Here's how the part is built. I have some questions about the finished solid (model axes, mm). Face numbers are marked on the shaded views. A direction names the side the tool comes from. Coordinates: 2 decimals unless noted, no trailing zeros. Write each loop counter-clockwise with the first axis right and the second up, starting at its lowest first coordinate (ties: lowest second). Pieces come first, ordered by that corner, then holes.
(1) Imagine slicing it at B-B, the plane z = -8.5. List the corners of the cut face in (x, y) for me, plus the area to 3 significant figures.
(2) Please list where these lines run through material, in increasing order: probe 1 along Y at (x, z) = (0, -6); probe 2 along X at (y, z) = (0, -9); probe 3 along X at (y, z) = (0, -7).
(3) Thinking about a two-plate mould opening in Y: for the marked faces 4, 5 and 6, which applies, released by +Y, released by -Y, zero draft, split by the parting line, or undercut?
(4) Which directions (+Z, -Z, +X, -X, +Y, -Y) give clear straight access to the entire face, cutting with the end or side of a thin tool? Please do the marked faces 1, 2 and 3.
(5) Imagine slicing it at A-A, the plane x = 0. List the corners of the cut face in (y, z) for me.
(6) For pin 1 Ø1 at (y, z) = (-4, -7.5) entering from +X; pin 2 Ø2 at (x, y) = (-3.5, 3) entering from +Z, each with a flat end and sliding along its axis, tell me the tip position at first contact or that it passes through.
(7) Imagine slicing it at C-C, the plane z = -1.5. List the corners of the cut face in (x, y) for me.
(8) Imagine slicing it at D-D, the plane z = -4.5. List the corners of the cut face in (x, y) for me, plus the area to 3 significant figures.
```python
from build123d import *

# Parameters (mm, degrees)
F1_R     = 9.1
F1_R_2   = 6.1
F2_DEPTH = 5
F3_DEPTH = 12
F3_TAPER = 12
F4_R     = 4.25
F4_R_2   = 2.75
F5_DEPTH = 10
F6_SIZE  = 2.5


with BuildPart() as f2:
    # F1 (on Top) → F2 (new body)
    with BuildSketch(Plane.XY):
        Circle(F1_R)
        Circle(F1_R_2, mode=Mode.SUBTRACT)
    extrude(amount=F2_DEPTH)

    # F1 (on Top) → F3 (join)
    with BuildSketch(Plane.XY):
        Circle(F1_R)
        Circle(F1_R_2, mode=Mode.SUBTRACT)
        Circle(F1_R_2)
    extrude(amount=-F3_DEPTH, taper=F3_TAPER)

    # F4 (on face) → F5 (cut)
    with BuildSketch(Plane(origin=(0, 0, -12), x_dir=(1, 0, 0), z_dir=(0, 0, -1))):
        Circle(F4_R)
        Circle(F4_R_2, mode=Mode.SUBTRACT)
    extrude(amount=-F5_DEPTH, mode=Mode.SUBTRACT)

    # F6
    f6_edges = [f2.edges().sort_by_distance(p)[0] for p in [
        (-9.1, 0, 5),
    ]]
    chamfer(f6_edges, length=F6_SIZE)


solid = f2.part
```
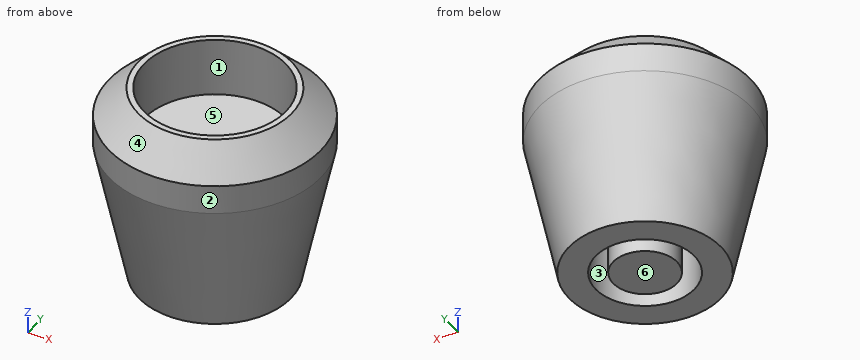
Recorded:
1. outline: circle Ø14.59 at (0, 0); circle Ø5.5 at (0, 0); hole circle Ø8.5 at (0, 0)
1. area: 134 mm2
2. probe 1: y = -7.82 to -4.25, -2.75 to 2.75, 4.25 to 7.82
2. probe 2: x = -7.19 to -4.25, -2.75 to 2.75, 4.25 to 7.19
2. probe 3: x = -7.61 to -4.25, -2.75 to 2.75, 4.25 to 7.61
3. face 4: split by the parting line
3. face 5: undercut
3. face 6: zero draft
4. face 1: +Z
4. face 2: +Z, -Z
4. face 3: -Z
5. outline: (-9.1, 0) - (-6.55, -12) - (-4.25, -12) - (-4.25, -2) - (-2.75, -2) - (-2.75, -12) - (2.75, -12) - (2.75, -2) - (4.25, -2) - (4.25, -12) - (6.55, -12) - (9.1, 0) - (9.1, 2.5) - (6.6, 5) - (6.1, 5) - (6.1, 0) - (-6.1, 0) - (-6.1, 5) - (-6.6, 5) - (-9.1, 2.5) - close
6. pin 1: stops at x = 6.67
6. pin 2: stops at z = 0
7. outline: circle Ø17.56 at (0, 0)
8. outline: circle Ø16.29 at (0, 0); circle Ø5.5 at (0, 0); hole circle Ø8.5 at (0, 0)
8. area: 175 mm2
